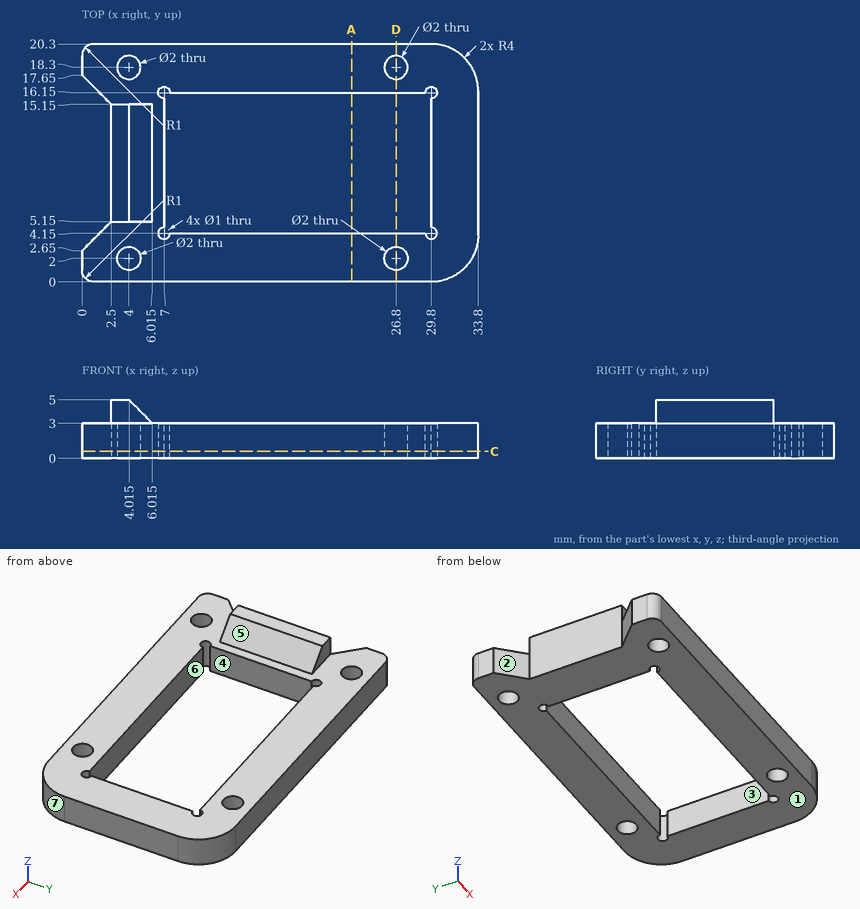
Job drawing, mm, ordinate dimensions from the low corner. One solid piece. A direction names the side the tool comes from. Coordinates: 2 decimals unless noted, no trailing zeros. Loops run counter-clockwise (first coordinate to the right, second up) from the corner with the lowest first, then second, coordinate; pieces in that order, holes last. Notation, with made-up numbers: (36, 48.25) - (54, 48.25) arc R26 ccw to (54, 76.25) - close; hole circle Ø3 at (-8.75, 67). An arc over 180 degrees is marked (long way). Write item = value, one per line. Start each with the question number.
Q1. Flat gauge pins, fed straight in: pin 1 Ø2.5 at (y, z) = (9, 1.5) entering from -X; pin 2 Ø10 at (x, y) = (10.5, 8.5) entering from +Z (1 decimal); pin 3 Ø1.6 at (x, y) = (26.8, 2) entering from -Z; pin 4 Ø2.5 at (x, y) = (4, 18.3) entering from +Z. Where does each tip first touch, or does it go through?
Q2. Pull direction Y, two halves, no side cores. Call the marked faces 4, 5, 6 and 7: pulls with the +Y half, pulls with the -Y half, needs draft (parallel to the pull), parting line crosses it, or undercut.
Q3. Cut at C-C, the plane z = 0.6. List the corners of the cut face in (x, y), then the cut area to 3 significant figures.
Q4. Which spindle directions (+Z, -Z, +X, -X, +Y, -Y) get a long thin tool onto all of the face, cutting with end or side? Do the marked faces 1, 2 and 3. Say none if no direction does.
Q5. Cut at D-D, the plane x = 26.8. List the corners of the cut face in (y, z), then the cut area to 3 significant figures.
Q6. Cut at A-A, the plane x = 23. List the corners of the cut face in (y, z).
Q7. Drill centre lines: L1, parallel to Y at x = 4, z = 1.85; L2, parallel to X at y = 10, z = 0.8; L3, parallel to Y at x = 28, z = 0.55. Where is each one in solid material? Low to high.
Computed:
q1.pin_1 = 2.5
q1.pin_2 = 3.5
q1.pin_3 = through
q1.pin_4 = 3
q2.face_4 = undercut
q2.face_5 = needs draft
q2.face_6 = undercut
q2.face_7 = pulls with the -Y half
q3.outline = (0, 1) arc R1 ccw to (1, 0) - (29.8, 0) arc R4 ccw to (33.8, 4) - (33.8, 16.3) arc R4 ccw to (29.8, 20.3) - (1, 20.3) arc R1 ccw to (0, 19.3) - (0, 17.65) - (2.5, 15.15) - (2.5, 5.15) - (0, 2.65) - close; hole circle Ø2 at (4, 2); hole circle Ø2 at (4, 18.3); hole (7, 4.65) arc R0.5 ccw (long way) to (7.5, 4.15) - (29.3, 4.15) arc R0.5 ccw (long way) to (29.8, 4.65) - (29.8, 15.65) arc R0.5 ccw (long way) to (29.3, 16.15) - (7.5, 16.15) arc R0.5 ccw (long way) to (7, 15.65) - close; hole circle Ø2 at (26.8, 2); hole circle Ø2 at (26.8, 18.3)
q3.area = 359 mm²
q4.face_1 = -Z, +X, -X, +Y, -Y
q4.face_2 = +Z, -Z, -X
q4.face_3 = +Z, -Z
q5.outline = (0, 0) - (1, 0) - (1, 3) - (0, 3) - close; (3, 0) - (4.15, 0) - (4.15, 3) - (3, 3) - close; (16.15, 0) - (17.3, 0) - (17.3, 3) - (16.15, 3) - close; (19.3, 0) - (20.3, 0) - (20.3, 3) - (19.3, 3) - close
q5.area = 12.9 mm²
q6.outline = (0, 0) - (4.15, 0) - (4.15, 3) - (0, 3) - close; (16.15, 0) - (20.3, 0) - (20.3, 3) - (16.15, 3) - close
q7.L1 = 0 to 1, 3 to 17.3, 19.3 to 20.3
q7.L2 = 2.5 to 7, 29.8 to 33.8
q7.L3 = 0 to 4.15, 16.15 to 20.3
